from build123d import *

# Parameters (mm, degrees)
SKETCH_1_W                  = 20
SKETCH_1_H                  = 20
EXTRUDE_1_DEPTH             = 4
EXTRUDE_2_DEPTH             = 130
EXTRUDE_2_DEPTH_BACK        = 20
SKETCH_2_W                  = 20
SKETCH_2_H                  = 4
SKETCH_3_W                  = 4
SKETCH_3_H                  = 24
EXTRUDE_3_DEPTH             = 130
SKETCH_4_W                  = 20
SKETCH_4_H                  = 40
EXTRUDE_4_DEPTH             = 4
HOLE_WIZARD_M53_D           = 5.2
HOLE_WIZARD_M53_ON_FACE_2_D = 5.2
HOLE_WIZARD_M53_ON_FACE_3_D = 5.2
FILLET_1_R                  = 2.5


with BuildPart() as part:
    # Эскиз1 → Бобышка-Вытянуть1 (new body)
    with BuildSketch(Plane.XY):
        with Locations((10, 10)):
            Rectangle(SKETCH_1_W, SKETCH_1_H)
    extrude(amount=EXTRUDE_1_DEPTH)

    # Эскиз2 → Бобышка-Вытянуть2 (add, two sides: drawn at the far end of the back side and taken through both)
    with BuildSketch(Plane.XY.offset(-EXTRUDE_2_DEPTH_BACK)):
        with Locations((10, 22)):
            Rectangle(SKETCH_2_W, SKETCH_2_H)
    extrude(amount=EXTRUDE_2_DEPTH + EXTRUDE_2_DEPTH_BACK)

    # Эскиз3 → Бобышка-Вытянуть3 (add)
    with BuildSketch(Plane(origin=(0, 0, 0), x_dir=(-1, 0, 0), z_dir=(0, 0, -1))):
        with Locations((-18, 12)):
            Rectangle(SKETCH_3_W, SKETCH_3_H)
    extrude(amount=-EXTRUDE_3_DEPTH)

    # Эскиз4 → Бобышка-Вытянуть4 (add)
    with BuildSketch(Plane.XY.offset(130)):
        with Locations((10, 20)):
            Rectangle(SKETCH_4_W, SKETCH_4_H)
    extrude(amount=-EXTRUDE_4_DEPTH)

    # Отверстие с зазором M53 (through all)
    with Locations(Plane(origin=(10, 10, 4), x_dir=(1, 0, 0), z_dir=(0, 0, 1))):
        with Locations((0, 0)):
            Hole(HOLE_WIZARD_M53_D / 2)

    # Отверстие с зазором M53 on face 2 (through all)
    with Locations(Plane(origin=(10, 24, -10), x_dir=(0, 0, 1), z_dir=(0, 1, 0))):
        with Locations((0, 0)):
            Hole(HOLE_WIZARD_M53_ON_FACE_2_D / 2)

    # Отверстие с зазором M53 on face 3 (through all)
    with Locations(Plane(origin=(10, 30, 126), x_dir=(-1, 0, 0), z_dir=(0, 0, -1))):
        with Locations((0, 0), (0, -20)):
            Hole(HOLE_WIZARD_M53_ON_FACE_3_D / 2)

    # Скругление1
    fillet_1_edges = [part.edges().sort_by_distance(p)[0] for p in [
        (0, 22, -20),
        (20, 22, -20),
        (0, 0, 128),
        (20, 40, 128),
        (0, 40, 128),
        (0, 0, 2),
    ]]
    fillet(fillet_1_edges, radius=FILLET_1_R)


solid = part.part
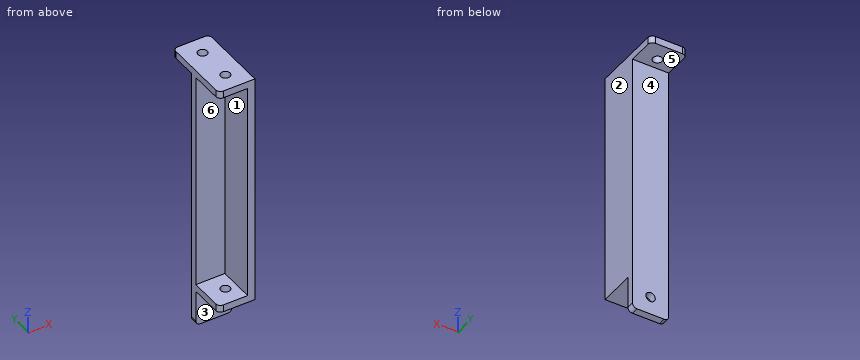
Check sheet for the modelled part. Datum: model origin and axes. Units: mm. Face numbers are marked on the shaded views. A direction names the side the tool comes from. Give positions to 0.01 mm unless a question says otherwise; leave off trailing zeros. Write each loop counter-clockwise with the first axis right and the second up, starting at its lowest first coordinate (ties: lowest second). Pieces come first, ordered by that corner, then holes. Notation, with made-up numbers: (35.25, -35.75) -> (51.25, -35.75) arc R22 ccw to (51.25, -21.75) -> close; hole circle Ø2 at (85.5, -31). An arc over 180 degrees is marked (long way). One line per item, written item: value. Start each with the question number.
Item 1: Section check A-A on y = 10. Record the cut outline in (x, z), then the cut area to 3 significant figures.
Item 2: Section check C-C on x = 10. Record the cut outline in (y, z), then the cut area to 3 significant figures.
Item 3: Material ranges on probe 1 along Y at (x, z) = (10, 129.2); probe 2 along X at (y, z) = (10, 2); probe 3 along Z at (x, y) = (5.25, 5), recorded low to high. Write a range as from..to.
Item 4: Tool access check on the marked faces 1, 2 and 3. Record the directions out of +Z, -Z, +X, -X, +Y, -Y that give a thin tool (end or side, any length) a straight path to the whole face; none if there is none.
Item 5: Gauge pin test, flat ends, axial feed: pin 1 (16 mm diameter, centred on y = 6.5, z = 41.5, fed in from -X); pin 2 (7 mm diameter, centred on x = 10, z = -10, fed in from -Y); pin 3 (8.5 mm diameter, centred on x = 10, y = 10, fed in from -Z). Record the tip position at first contact, or that the pin passes through.
Item 6: Section check B-B on z = -10. Record the cut outline in (x, y).
Item 7: Section check D-D on y = 30. Record the cut outline in (x, z).
Item 8: Draft check along Z on the marked faces 4, 5 and 6. Enter one of: +Z half, -Z half, draft (parallel to the pull), parting line (faces both ways), or undercut.
Results list:
1. outline: (0, 0) -> (7.4, 0) -> (7.4, 4) -> (0, 4) -> close; (0, 126) -> (7.4, 126) -> (7.4, 130) -> (0, 130) -> close; (12.6, 0) -> (20, 0) -> (20, 130) -> (12.6, 130) -> (12.6, 126) -> (16, 126) -> (16, 4) -> (12.6, 4) -> close
1. area: 606 mm²
2. outline: (0, 0) -> (7.4, 0) -> (7.4, 4) -> (0, 4) -> close; (0, 126) -> (7.4, 126) -> (7.4, 130) -> (0, 130) -> close; (12.6, 0) -> (20, 0) -> (20, -7.4) -> (24, -7.4) -> (24, 126) -> (27.4, 126) -> (27.4, 130) -> (12.6, 130) -> (12.6, 126) -> (20, 126) -> (20, 4) -> (12.6, 4) -> close; (20, -20) -> (24, -20) -> (24, -12.6) -> (20, -12.6) -> close; (32.6, 126) -> (40, 126) -> (40, 130) -> (32.6, 130) -> close
2. area: 741 mm²
3. probe 1: 0..7.4, 12.6..27.4, 32.6..40
3. probe 2: 0..7.4, 12.6..20
3. probe 3: 0..4, 126..130
4. face 1: -X, -Y
4. face 2: +Z, -Z, +X, +Y, -Y
4. face 3: -Z, +X, -X, -Y
5. pin 1: x = 16
5. pin 2: y = 20
5. pin 3: z = 0
6. outline: (0, 20) -> (7.4, 20) -> (7.4, 24) -> (0, 24) -> close; (12.6, 20) -> (20, 20) -> (20, 24) -> (12.6, 24) -> close
7. outline: (0, 126) -> (7.4, 126) -> (7.4, 130) -> (0, 130) -> close; (12.6, 126) -> (20, 126) -> (20, 130) -> (12.6, 130) -> close
8. face 4: draft
8. face 5: -Z half
8. face 6: undercut
